Input: dimensioned drawing with shaded views. Units: mm. Origin: part minimum x, y, z. A direction names the side the tool comes from. Coordinates: 2 decimals unless noted, no trailing zeros. Order: outer loops, then holes, each group sorted by start corner. A loop starts at its lowest first (then second) coordinate and runs counter-clockwise, first axis right, second up. Notation, with made-up numbers: (87.5, 36) -> (108.5, 36) arc R15 cw to (108.5, 48) -> close; hole circle Ø4 at (56, 29.5). An arc over 180 degrees is marked (long way). Answer as CSV lines item,"result".
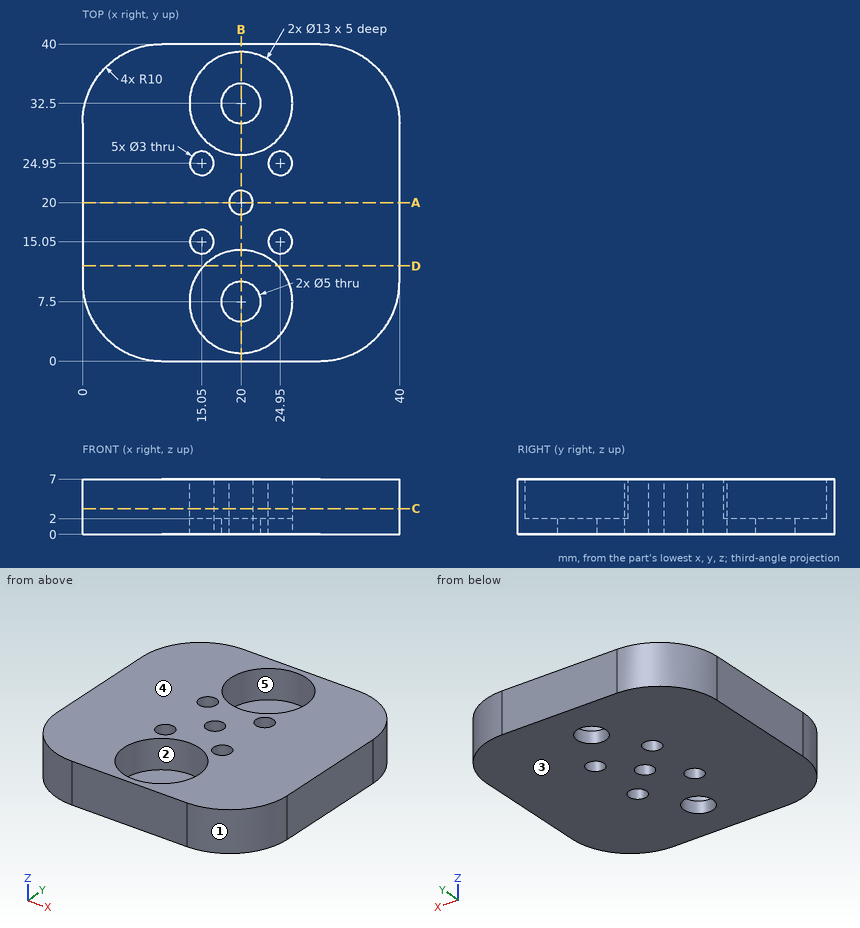
1. Ray query, line 1 along Y through (x, z) = (20, 5.4); line 2 along Y through (x, z) = (20, 1.2); line 3 along Z through (x, y) = (24, 7). Return the intervals inside material, ascending.
Findings:
line 1,"y = 0 to 1, 14 to 18.5, 21.5 to 26, 39 to 40"
line 2,"y = 0 to 5, 10 to 18.5, 21.5 to 30, 35 to 40"
line 3,"z = 0 to 2"
2. Cut plane A-A (y = 20). Return the cut outline in (x, z), plus the area to 3 significant figures.
Findings:
outline,"(0, 0) -> (18.5, 0) -> (18.5, 7) -> (0, 7) -> close; (21.5, 0) -> (40, 0) -> (40, 7) -> (21.5, 7) -> close"
area,"259 mm2"
3. Cut plane D-D (y = 12). Return the cut outline in (x, z).
Findings:
outline,"(0, 0) -> (40, 0) -> (40, 7) -> (24.69, 7) -> (24.69, 2) -> (15.31, 2) -> (15.31, 7) -> (0, 7) -> close"
4. Cut plane C-C (z = 3.25). Return the cut outline in (x, y).
Findings:
outline,"(0, 10) arc R10 ccw to (10, 0) -> (30, 0) arc R10 ccw to (40, 10) -> (40, 30) arc R10 ccw to (30, 40) -> (10, 40) arc R10 ccw to (0, 30) -> close; hole circle Ø13 at (20, 7.5); hole circle Ø13 at (20, 32.5); hole circle Ø3 at (15.05, 15.05); hole circle Ø3 at (15.05, 24.95); hole circle Ø3 at (20, 20); hole circle Ø3 at (24.95, 15.05); hole circle Ø3 at (24.95, 24.95)"
5. Reachability of the marked faces 4 and 5 from +Z, -Z, +X, -X, +Y, -Y: full face, straight path, thin tool, end or side. Return the list, or none.
Findings:
face 4,"+Z, +X, -X, +Y, -Y"
face 5,"+Z"
6. Contact query for flat-ended pins moving along their axis: pin 1 (3 mm diameter, centred on x = 20, y = 32.5, fed in from +Z); pin 2 (5 mm diameter, centred on x = 24.95, y = 24.95, fed in from -Z); pin 3 (4 mm diameter, centred on x = 5, z = 5.5, fed in from +Y); pin 4 (11.5 mm diameter, centred on x = 20, y = 7.5, fed in from +Z). Output: stop coordinate, or through.
Findings:
pin 1,"passes through"
pin 2,"stops at z = 0"
pin 3,"stops at y = 39.54"
pin 4,"stops at z = 2"
7. Cut plane B-B (x = 20). Return the cut outline in (y, z), plus the area to 3 significant figures.
Findings:
outline,"(0, 0) -> (5, 0) -> (5, 2) -> (1, 2) -> (1, 7) -> (0, 7) -> close; (10, 0) -> (18.5, 0) -> (18.5, 7) -> (14, 7) -> (14, 2) -> (10, 2) -> close; (21.5, 0) -> (30, 0) -> (30, 2) -> (26, 2) -> (26, 7) -> (21.5, 7) -> close; (35, 0) -> (40, 0) -> (40, 7) -> (39, 7) -> (39, 2) -> (35, 2) -> close"
area,"109 mm2"
8. Mould query, pull axis X, two halves, no side actions, for the marked faces 1, 2 and 3. Classes: released by +X, released by -X, zero draft, split by the parting line, or undercut.
Findings:
face 1,"released by +X"
face 2,"undercut"
face 3,"zero draft"
